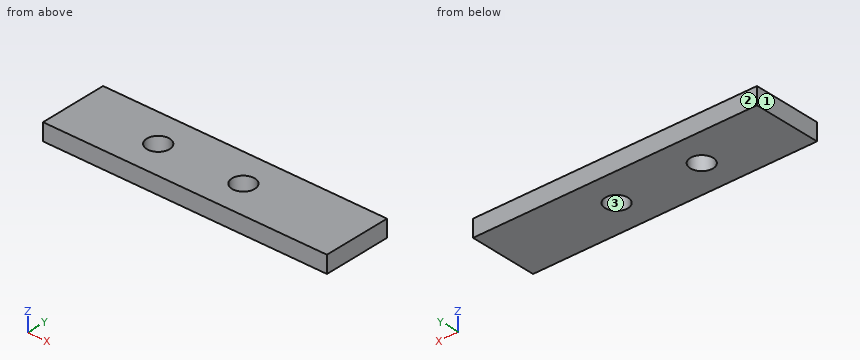
from build123d import *

# Parameters (mm, degrees)
PLAT_W                      = 60
PLAT_H                      = 15
EL_MENT_M_CANO_SOUD_1_DEPTH = 250
ESQUISSE2_R                 = 10
ENL_V_MAT_EXTRU_1_DEPTH     = 16


with BuildPart() as part:
    # plat → Elément mécano-soudé1 (new body)
    with BuildSketch(Plane.YZ):
        Rectangle(PLAT_W, PLAT_H)
    extrude(amount=EL_MENT_M_CANO_SOUD_1_DEPTH)

    # Esquisse2 → Enlèv. mat.-Extru.1 (cut, through all)
    with BuildSketch(Plane.XY.offset(7.5)):
        with Locations((150, 0)):
            Circle(ESQUISSE2_R)
        with Locations((75, 0)):
            Circle(ESQUISSE2_R)
    extrude(amount=-ENL_V_MAT_EXTRU_1_DEPTH, mode=Mode.SUBTRACT)


solid = part.part
Can you work these out from the model? Positions are in its coordinate system, mm. Face numbers are marked on the shaded views. Round coordinates to 2 decimals unless told otherwise and drop trailing zeros. Loops run counter-clockwise (first coordinate to the right, second up) from the corner with the lowest first, then second, coordinate; pieces in that order, holes last. Notation, with made-up numbers: (45.5, -24.5) - (89.5, -24.5) arc R26 ccw to (89.5, 13.5) - close; hole circle Ø2 at (4, 87). An arc over 180 degrees is marked (long way). Use CSV: the item, a comma, the result in double quotes. Start each with the question number.
1) If we section it at C-C on z = -3.5: Write out the boundary of the cut face in (x, y).
2) Please list where these lines run through material, in increasing order: probe 1 along X at (y, z) = (0.5, -2.5); probe 2 along Y at (x, z) = (75, -1); probe 3 along X at (y, z) = (-1, -4.5). Write a range as [from, to].
3) If we section it at B-B on x = 150: Write out the boundary of the cut face in (y, z).
4) If we section it at A-A on y = 0: Write out the boundary of the cut face in (x, z), plus the area to 3 significant figures.
5) We'd pull the mould along Y, two halves only. Please class the marked faces 1, 2 and 3: released by +Y, released by -Y, zero draft, split by the parting line, or undercut.
Geometry results:
1,outline,"(0, -30) - (250, -30) - (250, 30) - (0, 30) - close; hole circle Ø20 at (75, 0); hole circle Ø20 at (150, 0)"
2,probe 1,"x = [0, 65.01], [84.99, 140.01], [159.99, 250]"
2,probe 2,"y = [-30, -10], [10, 30]"
2,probe 3,"x = [0, 65.05], [84.95, 140.05], [159.95, 250]"
3,outline,"(-30, -7.5) - (-10, -7.5) - (-10, 7.5) - (-30, 7.5) - close; (10, -7.5) - (30, -7.5) - (30, 7.5) - (10, 7.5) - close"
4,outline,"(0, -7.5) - (65, -7.5) - (65, 7.5) - (0, 7.5) - close; (85, -7.5) - (140, -7.5) - (140, 7.5) - (85, 7.5) - close; (160, -7.5) - (250, -7.5) - (250, 7.5) - (160, 7.5) - close"
4,area,"3,150 mm2"
5,face 1,"zero draft"
5,face 2,"released by +Y"
5,face 3,"undercut"
